Study the drawing (mm; zero at the part's minimum x, y, z) and answer. A direction names the side the tool comes from. Coordinates: 2 decimals unless noted, no trailing zeros. Loops run counter-clockwise (first coordinate to the right, second up) from the corner with the lowest first, then second, coordinate; pieces in that order, holes last. Notation, with made-up numbers: (59, -11.75) - (67, -11.75) arc R25 ccw to (67, 27.25) - close; hole circle Ø4 at (-4.75, -39.75). An arc over 180 degrees is marked (long way). Use one line per item in the form item = value. Start each with the question number.
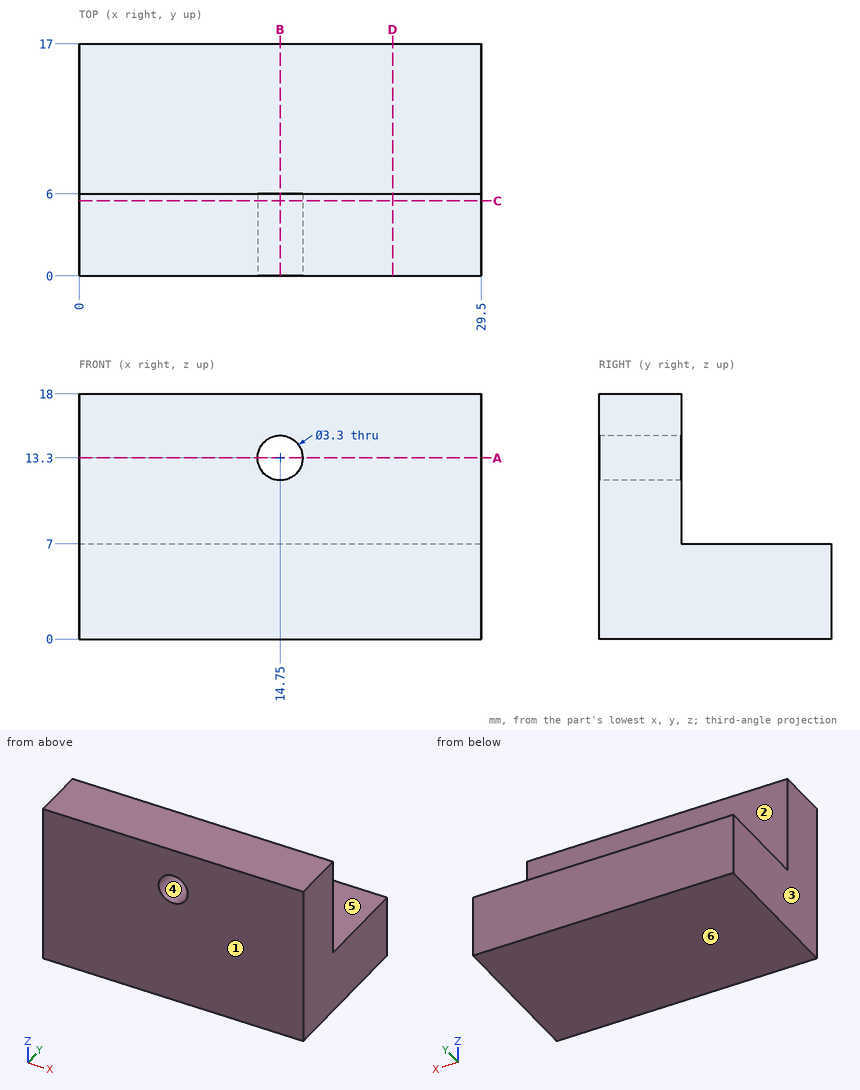
(1) A cutting plane is placed at A-A (z = 13.3). Determine the outline of the cut face in (x, y), then the cut area to 3 significant figures.
(2) Each of these flat-tipped pins is pushed along its axis until it touches: pin 1 Ø3 at (x, z) = (7.5, 16) entering from -Y; pin 2 Ø5.5 at (x, y) = (8, 13) entering from +Z; pin 3 Ø5.5 at (x, z) = (12, 12.5) entering from +Y. Where does it stop, or does it pass through?
(3) For the marked faces 1 and 2, determine the directions among +Z, -Z, +X, -X, +Y, -Y from which every point of the face is accessible in a straight line to the end or side of a thin tool.
(4) A cutting plane is placed at B-B (x = 14.75). Determine the outline of the cut face in (y, z).
(5) A cutting plane is placed at D-D (x = 23). Determine the outline of the cut face in (y, z).
(6) A cutting plane is placed at C-C (y = 5.5). Determine the outline of the cut face in (x, z), then the cut area to 3 significant figures.
(7) Determine the mould class of the marked faces 3, 4, 5 and 6 for opening direction Z: +Z half, -Z half, draft (parallel to the pull), parting line (faces both ways), or undercut.
(8) Find the intervals of material crossed by probe 1 along X at (y, z) = (3.65, 13.3); probe 2 along Z at (x, y) = (5, 6.75); probe 3 along Y at (x, z) = (6.25, 14.25), in increasing order. Write a range as from..to.
Evaluation:
q1.outline = (0, 0) - (13.1, 0) - (13.1, 6) - (0, 6) - close; (16.4, 0) - (29.5, 0) - (29.5, 6) - (16.4, 6) - close
q1.area = 157 mm^2
q2.pin_1 = 0
q2.pin_2 = 7
q2.pin_3 = 6
q3.face_1 = +Z, -Z, +X, -X, -Y
q3.face_2 = +Z, +X, -X, +Y
q4.outline = (0, 0) - (17, 0) - (17, 7) - (6, 7) - (6, 11.65) - (0, 11.65) - close; (0, 14.95) - (6, 14.95) - (6, 18) - (0, 18) - close
q5.outline = (0, 0) - (17, 0) - (17, 7) - (6, 7) - (6, 18) - (0, 18) - close
q6.outline = (0, 0) - (29.5, 0) - (29.5, 18) - (0, 18) - close; hole circle Ø3.3 at (14.75, 13.3)
q6.area = 522 mm^2
q7.face_3 = draft
q7.face_4 = undercut
q7.face_5 = +Z half
q7.face_6 = -Z half
q8.probe_1 = 0..13.1, 16.4..29.5
q8.probe_2 = 0..7
q8.probe_3 = 0..6
